Geometry check sheet. Reference: the model listing, model coordinates, mm. Round coordinates to 2 decimals unless told otherwise and drop trailing zeros. Loops run counter-clockwise (first coordinate to the right, second up) from the corner with the lowest first, then second, coordinate; pieces in that order, holes last. Notation, with made-up numbers: M 19.25,20 L 57.25,20 A23 ccw 57.25,31 Z; hole C 59.25,41.25 d8. An arc over 180 degrees is marked long. Use one line per item in the form item = value. Start each with the question number.
1. Draft check along Z on faces 1 (the cylindrical face through (19.566, -7.888, -20.857)), 2 (the flat face through (-1, 0, -47)), 3 (the flat face through (60.67, -7.89, -40.92)), 4 (the flat face through (-1, -8, -95)). Enter one of: pulls with the +Z half, pulls with the -Z half, needs draft (parallel to the pull), parting line crosses it, or undercut.
2. Cross-section at A-A (y = -11.5). Record the boundary of the cut face in (x, z).
3. Cross-section at C-C (z = -39). Record the boundary of the cut face in (x, y).
4. Go/stop test with flat-tipped pins: pin 1 (4 mm diameter, centred on x = 25.5, y = -6, fed in from +Z); pin 2 (1.5 mm diameter, centred on x = 36.5, y = -12, fed in from +Z); pin 3 (8 mm diameter, centred on x = 13.5, y = -3, fed in from +Z). Record where each tip stops, or that it passes through.
5. Cross-section at D-D (x = 65). Record the boundary of the cut face in (y, z), then the cut area to 3 significant figures.
6. Material ranges on line 1 (X direction, y = -11.5, z = -25); line 2 (X direction, y = -4.5, z = -8); line 3 (Z direction, x = -35, y = -3), recorded low to high.
7. Cross-section at B-B (z = -22.5). Record the boundary of the cut face in (x, y).
```python
from build123d import *

# Parameters (mm, degrees)
F1_DEPTH = 16


with BuildPart() as f1:
    # F0 (on Front) → F1 (new body)
    with BuildSketch(Plane.XZ):
        with BuildLine():
            ThreePointArc((18.330303, -17), (23.27292, -9.130784), (25, 0))
            ThreePointArc((25, 0), (23.774644, 7.730867), (20.218695, 14.70389))
            ThreePointArc((20.218695, 14.70389), (11.344663, 22.277761), (0, 25))
            ThreePointArc((0, 25), (-11.344663, 22.277761), (-20.218695, 14.70389))
            ThreePointArc((-20.218695, 14.70389), (-24.95577, -1.486451), (-18.330303, -17))
            ThreePointArc((-18.330303, -17), (-10.954451, -8.266799), (0, -5))
            ThreePointArc((0, -5), (10.954451, -8.266799), (18.330303, -17))
        make_face()
        with BuildLine():
            ThreePointArc((20.218695, 14.70389), (23.774644, 7.730867), (25, 0))
            ThreePointArc((25, 0), (23.27292, -9.130784), (18.330303, -17))
            ThreePointArc((18.330303, -17), (19.578126, -20.913807), (20, -25))
            ThreePointArc((20, -25), (-4.086193, -44.578126), (-18.330303, -17))
            ThreePointArc((-18.330303, -17), (-24.95577, -1.486451), (-20.218695, 14.70389))
            Line((-20.218695, 14.70389), (-100, -95))
            Line((-100, -95), (0, -95))
            Line((0, -95), (100, -95))
            Line((100, -95), (20.218695, 14.70389))
        make_face()
    extrude(amount=F1_DEPTH)


solid = f1.part
```
Reported:
q1.face_1 = undercut
q1.face_2 = needs draft
q1.face_3 = pulls with the +Z half
q1.face_4 = pulls with the -Z half
q2.outline = M -100,-95 L 100,-95 L 20.22,14.7 A25 ccw 0,25 A25 ccw -20.22,14.7 Z; hole M -18.33,-17 A20 ccw long 20,-25 A20 ccw 18.33,-17 A20 ccw 0,-5 A20 ccw Z
q3.outline = M -59.27,-16 L -14.28,-16 L -14.28,0 L -59.27,0 Z; M 14.28,-16 L 59.27,-16 L 59.27,0 L 14.28,0 Z
q4.pin_1 = 10.19
q4.pin_2 = -6.65
q4.pin_3 = 23.12
q5.outline = M -16,-95 L 0,-95 L 0,-46.87 L -16,-46.87 Z
q5.area = 770 mm²
q6.line_1 = -49.09 to -20, 20 to 49.09
q6.line_2 = -36.73 to -10.54, 10.54 to 36.73
q6.line_3 = -95 to -5.62
q7.outline = M -47.27,-16 L -19.84,-16 L -19.84,0 L -47.27,0 Z; M 19.84,-16 L 47.27,-16 L 47.27,0 L 19.84,0 Z
